from build123d import *

# Parameters (mm, degrees)
F0_W     = 1041.4
F0_H     = 914.4
F0_W_2   = 355.6
F0_H_2   = 12.7
F0_W_3   = 254
F1_DEPTH = 342.9


with BuildPart() as f1:
    # F0 (on Front) → F1 (new body)
    with BuildSketch(Plane.XZ):
        with Locations((31.582896, 242.074349)):
            Rectangle(F0_W, F0_H)
        Polygon((533.232896, -119.875651), (533.232896, -196.075651), (279.232896, -196.075651), (260.182896, -196.075651), (-95.417104, -196.075651), (-114.467104, -196.075651), (-470.067104, -196.075651), (-470.067104, -119.875651), (-470.067104, -107.175651), (-470.067104, -5.575651), (-470.067104, 7.124349), (-470.067104, 108.724349), (-470.067104, 121.424349), (-470.067104, 223.024349), (-470.067104, 235.724349), (-470.067104, 337.324349), (-470.067104, 350.024349), (-470.067104, 451.624349), (-470.067104, 464.324349), (-470.067104, 559.574349), (-470.067104, 565.924349), (-470.067104, 578.624349), (-470.067104, 680.224349), (-114.467104, 680.224349), (-95.417104, 680.224349), (260.182896, 680.224349), (279.232896, 680.224349), (533.232896, 680.224349), (533.232896, 578.624349), (533.232896, 565.924349), (533.232896, 464.324349), (533.232896, 451.624349), (533.232896, 350.024349), (533.232896, 337.324349), (533.232896, 235.724349), (533.232896, 223.024349), (533.232896, 121.424349), (533.232896, 108.724349), (533.232896, 7.124349), (533.232896, -5.575651), (533.232896, -107.175651), align=None, mode=Mode.SUBTRACT)
        Polygon((-470.067104, 559.574349), (-114.467104, 559.574349), (-114.467104, 565.924349), (-114.467104, 578.624349), (-470.067104, 578.624349), (-470.067104, 565.924349), align=None)
        Polygon((-114.467104, -196.075651), (-95.417104, -196.075651), (-95.417104, -119.875651), (-95.417104, -107.175651), (-95.417104, -5.575651), (-95.417104, 7.124349), (-95.417104, 108.724349), (-95.417104, 121.424349), (-95.417104, 223.024349), (-95.417104, 235.724349), (-95.417104, 337.324349), (-95.417104, 350.024349), (-95.417104, 451.624349), (-95.417104, 464.324349), (-95.417104, 565.924349), (-95.417104, 578.624349), (-95.417104, 680.224349), (-114.467104, 680.224349), (-114.467104, 578.624349), (-114.467104, 565.924349), (-114.467104, 559.574349), (-114.467104, 464.324349), (-114.467104, 451.624349), (-114.467104, 350.024349), (-114.467104, 337.324349), (-114.467104, 235.724349), (-114.467104, 223.024349), (-114.467104, 121.424349), (-114.467104, 108.724349), (-114.467104, 7.124349), (-114.467104, -5.575651), (-114.467104, -107.175651), (-114.467104, -119.875651), align=None)
        Polygon((260.182896, -196.075651), (279.232896, -196.075651), (279.232896, -119.875651), (279.232896, -107.175651), (279.232896, -5.575651), (279.232896, 7.124349), (279.232896, 108.724349), (279.232896, 121.424349), (279.232896, 223.024349), (279.232896, 235.724349), (279.232896, 337.324349), (279.232896, 350.024349), (279.232896, 451.624349), (279.232896, 464.324349), (279.232896, 565.924349), (279.232896, 578.624349), (279.232896, 680.224349), (260.182896, 680.224349), (260.182896, 578.624349), (260.182896, 565.924349), (260.182896, 464.324349), (260.182896, 451.624349), (260.182896, 350.024349), (260.182896, 337.324349), (260.182896, 235.724349), (260.182896, 223.024349), (260.182896, 121.424349), (260.182896, 108.724349), (260.182896, 7.124349), (260.182896, -5.575651), (260.182896, -107.175651), (260.182896, -119.875651), align=None)
        with Locations((82.382896, 572.274349)):
            Rectangle(F0_W_2, F0_H_2)
        with Locations((406.232896, 572.274349)):
            Rectangle(F0_W_3, F0_H_2)
        with Locations((406.232896, 457.974349)):
            Rectangle(F0_W_3, F0_H_2)
        with Locations((82.382896, 457.974349)):
            Rectangle(F0_W_2, F0_H_2)
        with Locations((-292.267104, 457.974349)):
            Rectangle(F0_W_2, F0_H_2)
        with Locations((-292.267104, 343.674349)):
            Rectangle(F0_W_2, F0_H_2)
        with Locations((-292.267104, 115.074349)):
            Rectangle(F0_W_2, F0_H_2)
        with Locations((-292.267104, 0.774349)):
            Rectangle(F0_W_2, F0_H_2)
        with Locations((-292.267104, -113.525651)):
            Rectangle(F0_W_2, F0_H_2)
        with Locations((82.382896, -113.525651)):
            Rectangle(F0_W_2, F0_H_2)
        with Locations((82.382896, 0.774349)):
            Rectangle(F0_W_2, F0_H_2)
        with Locations((82.382896, 115.074349)):
            Rectangle(F0_W_2, F0_H_2)
        with Locations((82.382896, 343.674349)):
            Rectangle(F0_W_2, F0_H_2)
        with Locations((82.382896, 229.374349)):
            Rectangle(F0_W_2, F0_H_2)
        with Locations((406.232896, 343.674349)):
            Rectangle(F0_W_3, F0_H_2)
        with Locations((406.232896, 229.374349)):
            Rectangle(F0_W_3, F0_H_2)
        with Locations((406.232896, 115.074349)):
            Rectangle(F0_W_3, F0_H_2)
        with Locations((406.232896, 0.774349)):
            Rectangle(F0_W_3, F0_H_2)
        with Locations((406.232896, -113.525651)):
            Rectangle(F0_W_3, F0_H_2)
        with Locations((-292.267104, 229.374349)):
            Rectangle(F0_W_2, F0_H_2)
    extrude(amount=-F1_DEPTH)


solid = f1.part
Model file for the job. Use its own axes, mm. A direction names the side the tool comes from. Give positions to 0.01 mm unless a question says otherwise; leave off trailing zeros. Loops run counter-clockwise (first coordinate to the right, second up) from the corner with the lowest first, then second, coordinate; pieces in that order, holes last.
Item 1: Which spindle directions (+Z, -Z, +X, -X, +Y, -Y) get a long thin tool onto all of the face, cutting with end or side? Do faces 1 (the face through (-9, 342.9, 346)), 2 (the face through (404, 169, 121.424)). Say none if no direction does.
Check values:
face 1: +Z, -Z, +X, -X, +Y
face 2: +Y, -Y
Item 2: Drill centre line: line 1 along X through (y, z) = (229, 466.5). Where is it in solid material? Low to high.
Check values:
line 1: x = -489.12 to -470.07, -114.47 to -95.42, 260.18 to 279.23, 533.23 to 552.28
Item 3: Slice it at B-B (x = -183). Give the number of separate pieces and of enclosed holes in the cut face, plus the area to 3 significant figures.
Check values:
separate pieces: 9
enclosed holes: 0
area: 45,700 mm2
Item 4: Mould opens along X. For faces 3 (the face through (-9, 0, 346)), 4 (the face through (-470.067, 169, 286)) say: +X half, -X half, draft (parallel to the pull), parting line (faces both ways), or undercut.
Check values:
face 3: draft
face 4: undercut
Item 5: Slice it at A-A (z = 418). Write the cut outline in (x, y).
Check values:
outline: (-489.12, 0) - (-470.07, 0) - (-470.07, 342.9) - (-489.12, 342.9) - close; (-114.47, 0) - (-95.42, 0) - (-95.42, 342.9) - (-114.47, 342.9) - close; (260.18, 0) - (279.23, 0) - (279.23, 342.9) - (260.18, 342.9) - close; (533.23, 0) - (552.28, 0) - (552.28, 342.9) - (533.23, 342.9) - close
